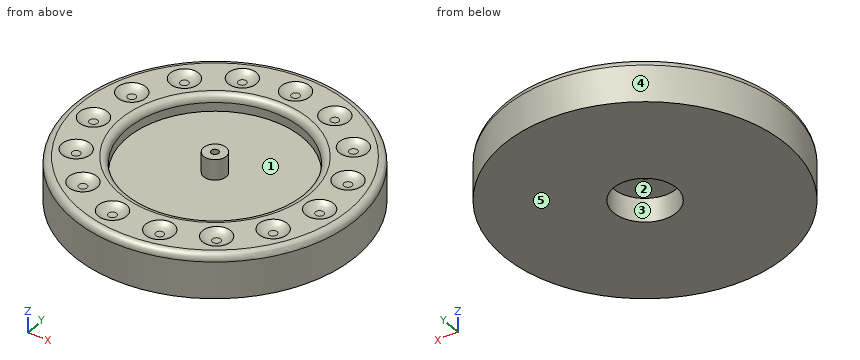
```python
from build123d import *

# Parameters (mm, degrees)
F0_R      = 50
F1_DEPTH  = 15.5
F2_R      = 31
F3_DEPTH  = 7.1
F4_R      = 11.125
F5_DEPTH  = 9
F6_R      = 2.5
F7_R      = 5
F8_DEPTH  = 1.5
F10_R     = 31.0625
F11_DEPTH = 1.5
F12_R     = 4
F13_DEPTH = 7.25
F15_D     = 2.65
F15_DEPTH = 10
F15_TIP   = 0.7961403202


# Not quite as in the source:
# - a fillet or chamfer that OpenCascade refuses, or shapes differently, is made with other operations: its cross-section is extruded or revolved along the edge and cut away or added


with BuildPart() as f1:
    # F0 (on Top) → F1 (new body)
    with BuildSketch(Plane.XY):
        Circle(F0_R)
    extrude(amount=F1_DEPTH)

    # F2 (on face) → F3 (cut)
    with BuildSketch(Plane.XY.offset(15.5)):
        Circle(F2_R)
    extrude(amount=-F3_DEPTH, mode=Mode.SUBTRACT)

    # F4 (on face) → F5 (cut)
    with BuildSketch(Plane.XY.offset(8.4)):
        Circle(F4_R)
    extrude(amount=-F5_DEPTH, mode=Mode.SUBTRACT)

    # F6
    f6_edges = [f1.edges().sort_by_distance(p)[0] for p in [
        (-50, 0, 15.5),
        (-31, 0, 15.5),
    ]]
    fillet(f6_edges, radius=F6_R)

    # F7 (on face) → F8 (cut)
    with BuildSketch(Plane.XY.offset(15.5)):
        with Locations((0, 40.5)):
            Circle(F7_R)
        with Locations((-16.4728340446, 36.9985910345)):
            Circle(F7_R)
        with Locations((-30.0973654318, 27.0997895575)):
            Circle(F7_R)
        with Locations((-38.51778891, 12.5151882722)):
            Circle(F7_R)
        with Locations((-40.2781367624, -4.2334027623)):
            Circle(F7_R)
        with Locations((-35.0740288533, -20.25)):
            Circle(F7_R)
        with Locations((-23.8053027178, -32.7651882722)):
            Circle(F7_R)
        with Locations((-8.4204234781, -39.6149778297)):
            Circle(F7_R)
        with Locations((8.4204234781, -39.6149778297)):
            Circle(F7_R)
        with Locations((23.8053027178, -32.7651882722)):
            Circle(F7_R)
        with Locations((35.0740288533, -20.25)):
            Circle(F7_R)
        with Locations((40.2781367624, -4.2334027623)):
            Circle(F7_R)
        with Locations((38.51778891, 12.5151882722)):
            Circle(F7_R)
        with Locations((30.0973654318, 27.0997895575)):
            Circle(F7_R)
        with Locations((16.4728340446, 36.9985910345)):
            Circle(F7_R)
    extrude(amount=-F8_DEPTH, mode=Mode.SUBTRACT)

    # F9: fillet of radius 5 on 15 edges, made by hand

    # F9_s1 → F9_t2 (revolve)
    with BuildSketch(Plane.XZ.offset(-40.5)):
        with BuildLine():
            ThreePointArc((5, 15.5), (3.3657774588, 14.3902277714), (1.4292857857, 14))
            Line((1.4292857857, 14), (5, 14))
            Line((5, 14), (5, 15.5))
        make_face()
    revolve(axis=Axis((0, 40.5, 14), (0, 0, 1)))

    # F9_s3 → F9_t4 (revolve)
    with BuildSketch(Plane.XZ.offset(-36.9985910345)):
        with BuildLine():
            ThreePointArc((-11.4728340446, 15.5), (-13.1070565857, 14.3902277714), (-15.0435482588, 14))
            Line((-15.0435482588, 14), (-11.4728340446, 14))
            Line((-11.4728340446, 14), (-11.4728340446, 15.5))
        make_face()
    revolve(axis=Axis((-16.4728340446, 36.9985910345, 14), (0, 0, 1)))

    # F9_s5 → F9_t6 (revolve)
    with BuildSketch(Plane.XZ.offset(-27.0997895575)):
        with BuildLine():
            ThreePointArc((-25.0973654318, 15.5), (-26.731587973, 14.3902277714), (-28.6680796461, 14))
            Line((-28.6680796461, 14), (-25.0973654318, 14))
            Line((-25.0973654318, 14), (-25.0973654318, 15.5))
        make_face()
    revolve(axis=Axis((-30.0973654318, 27.0997895575, 14), (0, 0, 1)))

    # F9_s7 → F9_t8 (revolve)
    with BuildSketch(Plane.XZ.offset(-12.5151882722)):
        with BuildLine():
            ThreePointArc((-33.51778891, 15.5), (-35.1520114511, 14.3902277714), (-37.0885031242, 14))
            Line((-37.0885031242, 14), (-33.51778891, 14))
            Line((-33.51778891, 14), (-33.51778891, 15.5))
        make_face()
    revolve(axis=Axis((-38.51778891, 12.5151882722, 14), (0, 0, 1)))

    # F9_s9 → F9_t10 (revolve)
    with BuildSketch(Plane.XZ.offset(4.2334027623)):
        with BuildLine():
            ThreePointArc((-35.2781367624, 15.5), (-36.9123593036, 14.3902277714), (-38.8488509767, 14))
            Line((-38.8488509767, 14), (-35.2781367624, 14))
            Line((-35.2781367624, 14), (-35.2781367624, 15.5))
        make_face()
    revolve(axis=Axis((-40.2781367624, -4.2334027623, 14), (0, 0, 1)))

    # F9_s11 → F9_t12 (revolve)
    with BuildSketch(Plane.XZ.offset(20.25)):
        with BuildLine():
            ThreePointArc((-30.0740288533, 15.5), (-31.7082513944, 14.3902277714), (-33.6447430675, 14))
            Line((-33.6447430675, 14), (-30.0740288533, 14))
            Line((-30.0740288533, 14), (-30.0740288533, 15.5))
        make_face()
    revolve(axis=Axis((-35.0740288533, -20.25, 14), (0, 0, 1)))

    # F9_s13 → F9_t14 (revolve)
    with BuildSketch(Plane.XZ.offset(32.7651882722)):
        with BuildLine():
            ThreePointArc((-18.8053027178, 15.5), (-20.439525259, 14.3902277714), (-22.3760169321, 14))
            Line((-22.3760169321, 14), (-18.8053027178, 14))
            Line((-18.8053027178, 14), (-18.8053027178, 15.5))
        make_face()
    revolve(axis=Axis((-23.8053027178, -32.7651882722, 14), (0, 0, 1)))

    # F9_s15 → F9_t16 (revolve)
    with BuildSketch(Plane.XZ.offset(39.6149778297)):
        with BuildLine():
            ThreePointArc((-3.4204234781, 15.5), (-5.0546460193, 14.3902277714), (-6.9911376924, 14))
            Line((-6.9911376924, 14), (-3.4204234781, 14))
            Line((-3.4204234781, 14), (-3.4204234781, 15.5))
        make_face()
    revolve(axis=Axis((-8.4204234781, -39.6149778297, 14), (0, 0, 1)))

    # F9_s17 → F9_t18 (revolve)
    with BuildSketch(Plane.XZ.offset(39.6149778297)):
        with BuildLine():
            ThreePointArc((13.4204234781, 15.5), (11.786200937, 14.3902277714), (9.8497092638, 14))
            Line((9.8497092638, 14), (13.4204234781, 14))
            Line((13.4204234781, 14), (13.4204234781, 15.5))
        make_face()
    revolve(axis=Axis((8.4204234781, -39.6149778297, 14), (0, 0, 1)))

    # F9_s19 → F9_t20 (revolve)
    with BuildSketch(Plane.XZ.offset(32.7651882722)):
        with BuildLine():
            ThreePointArc((28.8053027178, 15.5), (27.1710801767, 14.3902277714), (25.2345885036, 14))
            Line((25.2345885036, 14), (28.8053027178, 14))
            Line((28.8053027178, 14), (28.8053027178, 15.5))
        make_face()
    revolve(axis=Axis((23.8053027178, -32.7651882722, 14), (0, 0, 1)))

    # F9_s21 → F9_t22 (revolve)
    with BuildSketch(Plane.XZ.offset(20.25)):
        with BuildLine():
            ThreePointArc((40.0740288533, 15.5), (38.4398063121, 14.3902277714), (36.503314639, 14))
            Line((36.503314639, 14), (40.0740288533, 14))
            Line((40.0740288533, 14), (40.0740288533, 15.5))
        make_face()
    revolve(axis=Axis((35.0740288533, -20.25, 14), (0, 0, 1)))

    # F9_s23 → F9_t24 (revolve)
    with BuildSketch(Plane.XZ.offset(4.2334027623)):
        with BuildLine():
            ThreePointArc((45.2781367624, 15.5), (43.6439142212, 14.3902277714), (41.7074225481, 14))
            Line((41.7074225481, 14), (45.2781367624, 14))
            Line((45.2781367624, 14), (45.2781367624, 15.5))
        make_face()
    revolve(axis=Axis((40.2781367624, -4.2334027623, 14), (0, 0, 1)))

    # F9_s25 → F9_t26 (revolve)
    with BuildSketch(Plane.XZ.offset(-12.5151882722)):
        with BuildLine():
            ThreePointArc((43.51778891, 15.5), (41.8835663688, 14.3902277714), (39.9470746957, 14))
            Line((39.9470746957, 14), (43.51778891, 14))
            Line((43.51778891, 14), (43.51778891, 15.5))
        make_face()
    revolve(axis=Axis((38.51778891, 12.5151882722, 14), (0, 0, 1)))

    # F9_s27 → F9_t28 (revolve)
    with BuildSketch(Plane.XZ.offset(-27.0997895575)):
        with BuildLine():
            ThreePointArc((35.0973654318, 15.5), (33.4631428907, 14.3902277714), (31.5266512176, 14))
            Line((31.5266512176, 14), (35.0973654318, 14))
            Line((35.0973654318, 14), (35.0973654318, 15.5))
        make_face()
    revolve(axis=Axis((30.0973654318, 27.0997895575, 14), (0, 0, 1)))

    # F9_s29 → F9_t30 (revolve)
    with BuildSketch(Plane.XZ.offset(-36.9985910345)):
        with BuildLine():
            ThreePointArc((21.4728340446, 15.5), (19.8386115034, 14.3902277714), (17.9021198303, 14))
            Line((17.9021198303, 14), (21.4728340446, 14))
            Line((21.4728340446, 14), (21.4728340446, 15.5))
        make_face()
    revolve(axis=Axis((16.4728340446, 36.9985910345, 14), (0, 0, 1)))

    # F10 (on face) → F11 (join)
    with BuildSketch(Plane.XY.offset(8.4)):
        Circle(F10_R)
    extrude(amount=F11_DEPTH)

    # F12 (on face) → F13 (join)
    with BuildSketch(Plane.XY.offset(9.9)):
        Circle(F12_R)
    extrude(amount=F13_DEPTH)

    # F15
    with Locations(Plane.XY.offset(17.15)):
        with Locations((0, 0)):
            Hole(F15_D / 2, depth=F15_DEPTH)
            with Locations((0, 0, -(F15_DEPTH + F15_TIP / 2))):  # 118° drill point
                Cone(0, F15_D / 2, F15_TIP, mode=Mode.SUBTRACT)


solid = f1.part
```
Can you work these out from the model? Positions are in its coordinate system, mm. Face numbers are marked on the shaded views. A direction names the side the tool comes from. Round coordinates to 2 decimals unless told otherwise and drop trailing zeros. Loops run counter-clockwise (first coordinate to the right, second up) from the corner with the lowest first, then second, coordinate; pieces in that order, holes last. Notation, with made-up numbers: (85.5, 37.25) -> (114.5, 37.25) arc R25 cw to (114.5, 74.25) -> close; hole circle Ø3 at (75, 35). An arc over 180 degrees is marked (long way). Answer in a Markdown table with one row per item.
Item 1: On a 3-axis mill with a long thin cutter (end or side, diameter ignored), from which of +Z, -Z, +X, -X, +Y, -Y can I reach the whole of each face in a straight line? I mean the marked faces 1 and 2. Say none if no direction works.
Answer block:
| item | result |
|---|---|
| face 1 | +Z |
| face 2 | -Z |
Item 2: We'd pull the mould along X, two halves only. Please class the marked faces 3, 4 and 5: released by +X, released by -X, zero draft, split by the parting line, or undercut.
Answer block:
| item | result |
|---|---|
| face 3 | undercut |
| face 4 | split by the parting line |
| face 5 | zero draft |
Item 3: Suppose I cut it at A-A, the plane z = 6. List the corners of the cut face in (x, y) for me (3 decimals).
Answer block:
| item | result |
|---|---|
| outline | circle Ø100 at (0, 0); hole circle Ø22.25 at (0, 0) |
Item 4: Will these pins go through, and if not, where does the flat tip stop? P1, Ø0.9, axis at x = -16.5, y = 37.5, coming from the +Z side; P2, Ø1.5, axis at y = 9.5, z = 2.5, coming from the -X side; P3, Ø3, axis at x = -24.5, y = -33, coming from the +Z side; P4, Ø1.5, axis at x = -38, y = -19, coming from the -Z side.
Answer block:
| item | result |
|---|---|
| P1 | z = 14 |
| P2 | x = -49.23 |
| P3 | z = 14.07 |
| P4 | z = 0 |
Item 5: If I drill on probe 1 along Y at (x, z) = (0, 12.15) (3 decimals); probe 2 along X at (y, z) = (13.5, 14.75); probe 3 along Z at (x, y) = (25, -38.5), over which ranges is the centre line in solid material (lowest first)?
Answer block:
| item | result |
|---|---|
| probe 1 | -50 to -31, -4 to -1.325, 1.325 to 4, 31 to 50 |
| probe 2 | -47.4 to -42.46, -34.58 to -28.7, 28.7 to 34.58, 42.46 to 47.4 |
| probe 3 | 0 to 15.5 |
